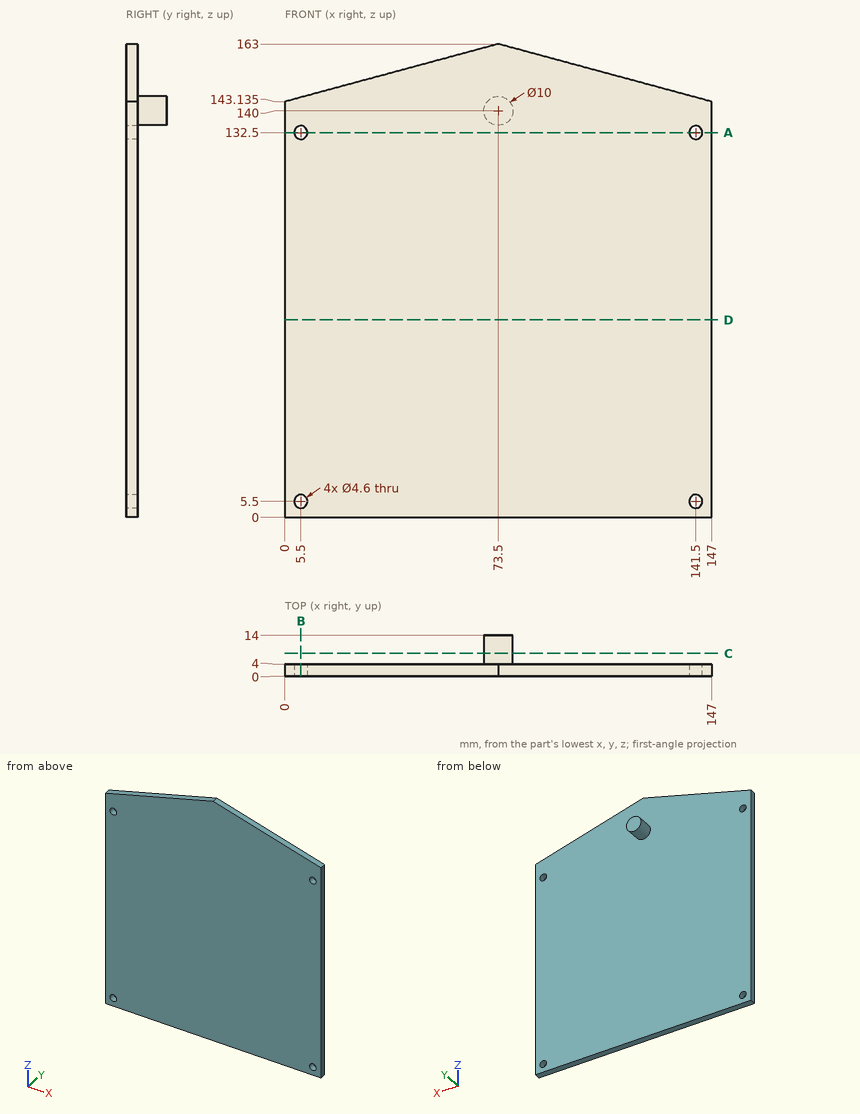
Verification items for this drawing (mm, ordinates from the low corner). Coordinates: 2 decimals unless noted, no trailing zeros. Order: outer loops, then holes, each group sorted by start corner. A loop starts at its lowest first (then second) coordinate and runs counter-clockwise, first axis right, second up. Notation, with made-up numbers: (-18.75, -25) - (-10.75, -25) arc R28 ccw to (-10.75, 1) - close; hole circle Ø7 at (18.5, 85.25). An arc over 180 degrees is marked (long way). Use one line per item in the form item = value.
1. Gauge pin test, flat end, axial feed: pin 1 (1 mm diameter, centred on x = 125.5, z = 125, fed in from +Y). Record the tip position at first contact, or that the pin passes through.
Here are the results:
pin_1 = 4
2. Section check D-D (z = 68). Record the boundary of the cut face in (x, y), then the cut area to 3 significant figures.
Here are the results:
outline = (0, 0) - (147, 0) - (147, 4) - (0, 4) - close
area = 588 mm²
3. Section check A-A (z = 132.5). Record the boundary of the cut face in (x, y), then the cut area to 3 significant figures.
Here are the results:
outline = (0, 0) - (3.2, 0) - (3.2, 4) - (0, 4) - close; (7.8, 0) - (139.2, 0) - (139.2, 4) - (7.8, 4) - close; (143.8, 0) - (147, 0) - (147, 4) - (143.8, 4) - close
area = 551 mm²
4. Section check B-B (x = 5.5). Record the boundary of the cut face in (y, z), then the cut area to 3 significant figures.
Here are the results:
outline = (0, 0) - (4, 0) - (4, 3.2) - (0, 3.2) - close; (0, 7.8) - (4, 7.8) - (4, 130.2) - (0, 130.2) - close; (0, 134.8) - (4, 134.8) - (4, 144.62) - (0, 144.62) - close
area = 542 mm²
5. Scan lines: line 1 (X direction, y = 1.2, z = 132.5); line 2 (Z direction, x = 5.5, y = 2.2); line 3 (Y direction, x = 60.5, z = 36.5). Record each from-to range of solid material in increasing order.
Here are the results:
line_1 = 0 to 3.2, 7.8 to 139.2, 143.8 to 147
line_2 = 0 to 3.2, 7.8 to 130.2, 134.8 to 144.62
line_3 = 0 to 4
6. Section check C-C (y = 7.75). Record the boundary of the cut face in (x, z).
Here are the results:
outline = circle Ø10 at (73.5, 140)
